Source: CAD feature listing. Evaluate the final solid. Frame: model axes, mm. Give positions to 0.01 mm unless a question says otherwise; leave off trailing zeros. Order: outer loops, then holes, each group sorted by start corner. A loop starts at its lowest first (then second) coordinate and runs counter-clockwise, first axis right, second up. Notation, with made-up numbers: M 14,6.25 L 47,6.25 A34 cw 47,39.25 Z; hole C 85.5,-35 d3. An arc over 180 degrees is marked long. Answer as a JSON object with one key per item and string values. Group by question number.
1. Pull-direction query (X, two-part tool) for faces 1 (the flat face through (-32, 2, 8.048)), 2 (the flat face through (-1, 2, 40.085)); classes: +X half, -X half, draft (parallel to the pull), parting line (faces both ways), or undercut.
2. Section query A-A (z = 21). Output: boundary loops of the cut face in (x, y) (3 decimals).
3. Section query B-B (y = 1.1). Count the separate pieces of the cut face and the enclosed holes in it, plus the area to 3 significant figures.
4. Material intervals for L1, parallel to X at y = 1.4, z = -12.5 (3 decimals), sorted ascending. Write a range as [from, to].
5. Pin query (flat end, axial travel): P1, Ø1.5, axis at x = -13, z = -2, coming from the -Y side. Return the tip coordinate at first contact, or that it passes through.
from build123d import *

# Parameters (mm, degrees)
SKETCH1_W           = 100.17
SKETCH1_H           = 80.17
BOSS_EXTRUDE1_DEPTH = 3.175
SKETCH2_W           = 6.08
SKETCH2_H           = 6.08
CUT_EXTRUDE2_DEPTH  = 4.175
LPATTERN1_COUNT     = 5
LPATTERN1_PITCH     = 11.0875
SKETCH4_R           = 1.415
CUT_EXTRUDE3_DEPTH  = 6.35


with BuildPart() as part:
    # Sketch1 → Boss-Extrude1 (new body)
    with BuildSketch(Plane(origin=(0, 0, 0), x_dir=(1, 0, 0), z_dir=(0, 1, 0))):
        Rectangle(SKETCH1_W, SKETCH1_H)
    extrude(amount=BOSS_EXTRUDE1_DEPTH)

    # Sketch2 → Cut-Extrude2 (cut, through all)
    with BuildSketch(Plane(origin=(0, 3.175, 0), x_dir=(1, 0, 0), z_dir=(0, 1, 0))):
        with Locations((-32.175, 22.175)):
            Rectangle(SKETCH2_W, SKETCH2_H)
        with Locations((32.175, 22.175)):
            Rectangle(SKETCH2_W, SKETCH2_H)
    cut_extrude2 = extrude(amount=-CUT_EXTRUDE2_DEPTH, mode=Mode.SUBTRACT)

    # LPattern1: Cut-Extrude2 ×5
    with Locations(*[(0, 0, i * LPATTERN1_PITCH) for i in range(1, LPATTERN1_COUNT)]):
        add(cut_extrude2, mode=Mode.SUBTRACT)

    # Sketch4 → Cut-Extrude3 (cut)
    with BuildSketch(Plane(origin=(0, 3.175, 0), x_dir=(1, 0, 0), z_dir=(0, 1, 0))):
        with Locations((-44.696699141, 34.696699141)):
            Circle(SKETCH4_R)
        with Locations((44.696699141, 34.696699141)):
            Circle(SKETCH4_R)
        with Locations((44.696699141, -34.696699141)):
            Circle(SKETCH4_R)
        with Locations((-44.696699141, -34.696699141)):
            Circle(SKETCH4_R)
    extrude(amount=-CUT_EXTRUDE3_DEPTH, mode=Mode.SUBTRACT)


solid = part.part
Answer sheet:
{
 "1": {"face 1": "undercut", "face 2": "draft"},
 "2": {"outline": "M -50.085,0 L -35.215,0 L -35.215,3.175 L -50.085,3.175 Z; M -29.135,0 L 29.135,0 L 29.135,3.175 L -29.135,3.175 Z; M 35.215,0 L 50.085,0 L 50.085,3.175 L 35.215,3.175 Z"},
 "3": {"separate pieces": "1", "enclosed holes": "14", "area": "7,640 mm^2"},
 "4": {"L1": "[-50.085, -35.215], [-29.135, 29.135], [35.215, 50.085]"},
 "5": {"P1": "y = 0"}
}
